Geometry: final body of the model. Coordinates: model frame, mm. A direction names the side the tool comes from. Give positions to 0.01 mm unless a question says otherwise; leave off trailing zeros. Loops run counter-clockwise (first coordinate to the right, second up) from the corner with the lowest first, then second, coordinate; pieces in that order, holes last. Notation, with made-up numbers: (5.5, -12.75) -> (52.5, -12.75) arc R11 cw to (52.5, 4.25) -> close; hole circle Ø5 at (68, -38). An arc over 180 degrees is marked (long way). Answer in a Markdown table with one row per item. Add a question column.
1) Section query A-A (x = 0). Return the cut outline in (y, z).
2) Section query C-C (z = 24.5). Return the cut outline in (x, y), plus the area to 3 significant figures.
3) Draft query along Y for faces 1 (the cylindrical face through (21.88, 23.073, 34.61)), 2 (the flat face through (22, 22, 70.1)). Return one class per face: +Y half, -Y half, draft (parallel to the pull), parting line (faces both ways), or undercut.
4) First-contact query: P1, Ø4, axis at y = 21, z = 32.5, coming from the -X side; P2, Ø12, axis at x = 19, z = 19, coming from the +Y side; P3, Ø21, axis at x = -5, y = -8, coming from the +Z side; P4, Ø12, axis at x = 15.5, z = 60, coming from the -Y side. Flat tips, straight axial feed; report the tip coordinate or a pass-through.
5) Line query: line 1 (Y direction, x = 23, z = 13). Output: solid intervals per line, ascending. Write a range as from..to.
6) Access query for faces 3 (the flat face through (-22, -22, 70.1)), 4 (the cylindrical face through (21.098, -22.141, 34.61)). Directions: +Z, -Z, +X, -X, +Y, -Y. A direction counts if a zero-diameter tool reaches every point of the face in a straight line with its end or side. Return the directions, or none.
Autodesk Inventor part; units mm, degrees
ref_plane "YZ Plane" through (0, 0, 0) normal (1, 0, 0) x (0, 1, 0)
ref_plane "XZ Plane" through (0, 0, 0) normal (0, 1, 0) x (-1, 0, 0)
ref_plane "XY Plane" through (0, 0, 0) normal (0, 0, 1) x (1, 0, 0)
sketch "Sketch1" plane through (0, 0, 0) normal (0, 0, 1) x (1, 0, 0)
  line L0 (-35, 35) -> (35, 35)
  line L1 (35, 35) -> (35, -35)
  line L2 (35, -35) -> (-35, -35)
  line L3 (-35, -35) -> (-35, 35)
  line L4 (-35, 35) -> (35, -35) construction
  line L5 (35, 35) -> (-35, -35) construction
  circle A0 centre (0, 0) radius 30
  dimension "d0" = 70
  dimension "d1" = 70
  dimension "d2" = 60
extrude "Extrusion1" add sketch "Sketch1" along normal blind 0.1
sketch "Sketch2" plane through (0, 0, 0.1) normal (0, 0, 1) x (1, 0, 0)
  circle A0 centre (-22.097, 22.097) radius 1
  circle A1 centre (22.097, 22.097) radius 1
  circle A2 centre (22.097, -22.097) radius 1
  circle A3 centre (-22.097, -22.097) radius 1
  line L0 (-35, 35) -> (-35, -35)
  line L1 (35, 35) -> (-35, 35)
  line L2 (35, -35) -> (35, 35)
  line L3 (-35, -35) -> (35, -35)
  point P0 (0, 0)
  dimension "d5" = 2
  dimension "d6" = 2
  dimension "d7" = 2
  dimension "d8" = 2
  dimension "d9" = 12.903
  dimension "d10" = 12.903
  dimension "d11" = 12.903
  dimension "d12" = 12.903
  dimension "d13" = 12.903
  dimension "d14" = 12.903
  dimension "d15" = 12.903
  dimension "d16" = 12.903
extrude "Extrusion2" add sketch "Sketch2" along normal blind 70 contours A0 | A1 | A2 | A3
properties part number "electrode_holder"
Evaluation:
| question | item | result |
|---|---|---|
| 1 | outline | (-35, 0) -> (-30, 0) -> (-30, 0.1) -> (-35, 0.1) -> close; (30, 0) -> (35, 0) -> (35, 0.1) -> (30, 0.1) -> close |
| 2 | outline | circle Ø2 at (-22.1, -22.1); circle Ø2 at (-22.1, 22.1); circle Ø2 at (22.1, -22.1); circle Ø2 at (22.1, 22.1) |
| 2 | area | 12.6 mm² |
| 3 | face 1 | undercut |
| 3 | face 2 | draft |
| 4 | P1 | x = -23.1 |
| 4 | P2 | y = 23.1 |
| 4 | P3 | through |
| 4 | P4 | y = -22.9 |
| 5 | line 1 | -22.53..-21.67, 21.67..22.53 |
| 6 | face 3 | +Z, +X, -X, +Y, -Y |
| 6 | face 4 | +Z |
